Verification items for this drawing (mm, ordinates from the low corner). Give positions to 0.01 mm unless a question says otherwise; leave off trailing zeros. Order: outer loops, then holes, each group sorted by start corner. A loop starts at its lowest first (then second) coordinate and runs counter-clockwise, first axis right, second up.
(1) Scan lines: L1, parallel to Z at x = 13.5, y = 4.25; L2, parallel to Y at x = 25.5, z = 10.75; L3, parallel to X at y = 6, z = 11.5. Record each from-to range of solid material in increasing order.
(2) Sectioned sample at D-D on x = 19.25. Record the cut outline in (y, z), plus the area to 3 significant figures.
(3) Sectioned sample at A-A on x = 13.5. Record the cut outline in (y, z).
(4) Sectioned sample at C-C on y = 4.25. Record the cut outline in (x, z).
(5) Mould release check, pull along Z, two halves, no side actions. Record for the marked faces 1, 2 and 3: pulls with the +Z half, pulls with the -Z half, needs draft (parallel to the pull), parting line crosses it, or undercut.
(6) Gauge pin test, flat ends, axial feed: pin 1 (1.5 mm diameter, centred on y = 6.5, z = 5, fed in from -X); pin 2 (1.5 mm diameter, centred on x = 15, z = 11, fed in from +Y) (3 decimals); pin 3 (13 mm diameter, centred on x = 13.5, z = 13.5, fed in from -Y); pin 4 (4 mm diameter, centred on y = 6.5, z = 14, fed in from -X). Record the tip position at first contact, or that the pin passes through.
(7) Sectioned sample at B-B on z = 13.5. Record the cut outline in (x, y), plus the area to 3 significant figures.
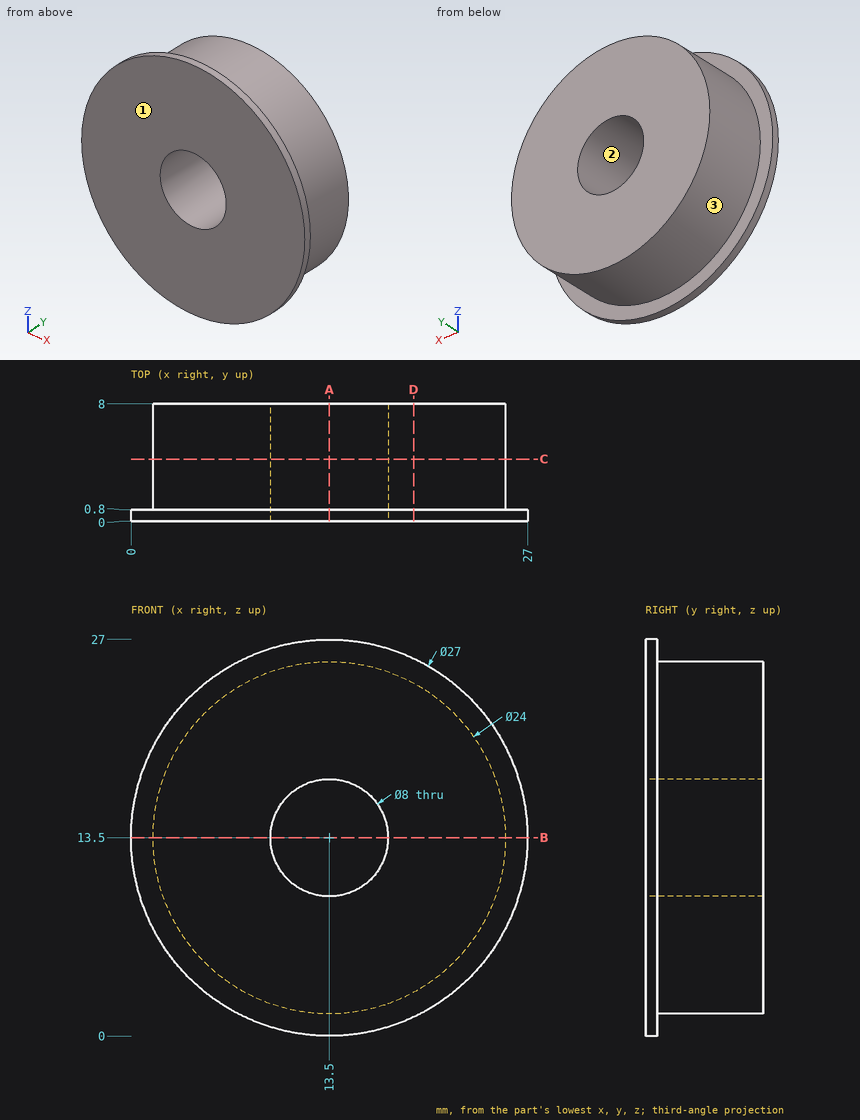
Ans:
1. L1: z = 1.5 to 9.5, 17.5 to 25.5
1. L2: y = 0 to 0.8
1. L3: x = 1.67 to 10.04, 16.96 to 25.33
2. outline: (0, 1.29) - (0.8, 1.29) - (0.8, 2.97) - (8, 2.97) - (8, 24.03) - (0.8, 24.03) - (0.8, 25.71) - (0, 25.71) - close
2. area: 171 mm2
3. outline: (0, 0) - (0.8, 0) - (0.8, 1.5) - (8, 1.5) - (8, 9.5) - (0, 9.5) - close; (0, 17.5) - (8, 17.5) - (8, 25.5) - (0.8, 25.5) - (0.8, 27) - (0, 27) - close
4. outline: circle Ø24 at (13.5, 13.5); hole circle Ø8 at (13.5, 13.5)
5. face 1: needs draft
5. face 2: undercut
5. face 3: parting line crosses it
6. pin 1: stops at x = 4.34
6. pin 2: passes through
6. pin 3: stops at y = 0
6. pin 4: stops at x = 1.5
7. outline: (0, 0) - (9.5, 0) - (9.5, 8) - (1.5, 8) - (1.5, 0.8) - (0, 0.8) - close; (17.5, 0) - (27, 0) - (27, 0.8) - (25.5, 0.8) - (25.5, 8) - (17.5, 8) - close
7. area: 130 mm2
